```python
from build123d import *

# Parameters (mm, degrees)
IZIM1_R                           = 40.225
Y_KSEKLIK_EKSTR_ZYON1_DEPTH       = 5
IZIM2_W                           = 5
IZIM2_H                           = 15
Y_KSEKLIK_EKSTR_ZYON2_DEPTH       = 64
IZIM3_W                           = 8.48037671
IZIM3_H                           = 5
KES_EKSTR_ZYON1_DEPTH             = 128
IZIM6_R                           = 25
Y_KSEKLIK_EKSTR_ZYON4_DEPTH       = 5
IZIM7_W                           = 5
IZIM7_H                           = 5
Y_KSEKLIK_EKSTR_ZYON5_DEPTH       = 2
IZIM8_W                           = 5
IZIM8_H                           = 5
Y_KSEKLIK_EKSTR_ZYON6_DEPTH       = 7
IZIM9_W                           = 5.33982185
IZIM9_H                           = 8.96327239
KES_EKSTR_ZYON2_DEPTH             = 23
IZIM10_W                          = 16.71
IZIM10_H                          = 5
Y_KSEKLIK_EKSTR_ZYON7_DEPTH       = 15
IZIM13_W                          = 0.39
IZIM13_H                          = 5
Y_KSEKLIK_EKSTR_ZYON9_DEPTH       = 15
Y_KSEKLIK_EKSTR_ZYON10_DEPTH      = 3
Y_KSEKLIK_EKSTR_ZYON10_DEPTH_BACK = 18
IZIM14_W                          = 15
IZIM14_H                          = 5
IZIM11_W                          = 15.71
IZIM11_H                          = 5
Y_KSEKLIK_EKSTR_ZYON11_DEPTH      = 15
Y_KSEKLIK_EKSTR_ZYON12_DEPTH      = 3
Y_KSEKLIK_EKSTR_ZYON12_DEPTH_BACK = 18
IZIM16_W                          = 15
IZIM16_H                          = 5
IZIM17_W                          = 120.128605811
IZIM17_H                          = 27.620146719
KES_EKSTR_ZYON3_DEPTH             = 50
IZIM18_R                          = 5
KES_EKSTR_ZYON4_DEPTH             = 100
IZIM20_R                          = 20
IZIM20_R_2                        = 10
Y_KSEKLIK_EKSTR_ZYON14_DEPTH      = 35
IZIM21_R                          = 10
KES_EKSTR_ZYON5_DEPTH             = 45


with BuildPart() as part:
    # Çizim1 → Yükseklik-Ekstrüzyon1 (new body)
    with BuildSketch(Plane.XY):
        Circle(IZIM1_R)
    extrude(amount=Y_KSEKLIK_EKSTR_ZYON1_DEPTH)

    # Çizim2 → Yükseklik-Ekstrüzyon2 (add, symmetric)
    with BuildSketch(Plane(origin=(0, 0, 0), x_dir=(0, 0, -1), z_dir=(1, 0, 0))):
        with Locations((-2.5, 0)):
            Rectangle(IZIM2_W, IZIM2_H)
    extrude(amount=Y_KSEKLIK_EKSTR_ZYON2_DEPTH, both=True)

    # Çizim3 → Kes-Ekstrüzyon1 (cut)
    with BuildSketch(Plane.XZ.offset(7.5)):
        with Locations((-59.759811645, 2.5)):
            Rectangle(IZIM3_W, IZIM3_H)
    extrude(amount=-KES_EKSTR_ZYON1_DEPTH, mode=Mode.SUBTRACT)

    # Çizim7 → Yükseklik-Ekstrüzyon5 (add)
    with BuildSketch(Plane.XY.offset(5)):
        Polygon((35.024990748, -17.334936491), (30.694863729, -14.834936491), (28.194863729, -19.165063509), (32.524990748, -21.665063509), align=None)
        with Locations((0, 36.5)):
            Rectangle(IZIM7_W, IZIM7_H)
        Polygon((-32.524990748, -21.665063509), (-28.194863729, -19.165063509), (-30.694863729, -14.834936491), (-35.024990748, -17.334936491), align=None)
    extrude(amount=Y_KSEKLIK_EKSTR_ZYON5_DEPTH)


with BuildPart() as body_2:
    # Çizim6 → Yükseklik-Ekstrüzyon4 (new body)
    with BuildSketch(Plane.XY.offset(25)):
        Circle(IZIM6_R)
    extrude(amount=Y_KSEKLIK_EKSTR_ZYON4_DEPTH)

    # Çizim8 → Yükseklik-Ekstrüzyon6 (add)
    with BuildSketch(Plane.XY.offset(30)):
        Polygon((22.034609691, -9.834936491), (17.704482672, -7.334936491), (15.204482672, -11.665063509), (19.534609691, -14.165063509), align=None)
        with Locations((0, 21.5)):
            Rectangle(IZIM8_W, IZIM8_H)
        Polygon((-19.534609691, -14.165063509), (-15.204482672, -11.665063509), (-17.704482672, -7.334936491), (-22.034609691, -9.834936491), align=None)
    extrude(amount=-Y_KSEKLIK_EKSTR_ZYON6_DEPTH)


    add(part.part)  # loft1 joins it to this body
    # loft from a face of the part (loft1)
    loft([body_2.faces().sort_by_distance((-18.619546181, -10.75, 23))[0], body_2.faces().sort_by_distance((-31.609927238, -18.25, 7))[0]])

    # loft from a face of the part (loft3)
    loft([body_2.faces().sort_by_distance((0, 36.5, 7))[0], body_2.faces().sort_by_distance((0, 21.5, 23))[0]])

    # Çizim9 → Kes-Ekstrüzyon2 (cut)
    with BuildSketch(Plane.XZ.offset(7.5)):
        with Locations((62.899534215, 2.077883617)):
            Rectangle(IZIM9_W, IZIM9_H)
    extrude(amount=-KES_EKSTR_ZYON2_DEPTH, mode=Mode.SUBTRACT)

    # Çizim10 → Yükseklik-Ekstrüzyon7 (add)
    with BuildSketch(Plane.XZ.offset(7.5)):
        with Locations((-52.87462329, 2.5)):
            Rectangle(IZIM10_W, IZIM10_H)
    extrude(amount=-Y_KSEKLIK_EKSTR_ZYON7_DEPTH)

    # Çizim13 → Yükseklik-Ekstrüzyon9 (add)
    with BuildSketch(Plane.XZ.offset(7.5)):
        with Locations((-61.42462329, 2.5)):
            Rectangle(IZIM13_W, IZIM13_H)
    extrude(amount=-Y_KSEKLIK_EKSTR_ZYON9_DEPTH)

    # Çizim14 → Yükseklik-Ekstrüzyon10 (add, two sides: drawn at the far end of the back side and taken through both)
    with BuildSketch(Plane.XZ.offset(7.5).offset(-Y_KSEKLIK_EKSTR_ZYON10_DEPTH_BACK)):
        with Locations((-53.40962329, 2.5)):
            Rectangle(IZIM14_W, IZIM14_H)
    extrude(amount=Y_KSEKLIK_EKSTR_ZYON10_DEPTH + Y_KSEKLIK_EKSTR_ZYON10_DEPTH_BACK)

    # Çizim11 → Yükseklik-Ekstrüzyon11 (add)
    with BuildSketch(Plane.XZ.offset(7.5)):
        with Locations((53.76462329, 2.5)):
            Rectangle(IZIM11_W, IZIM11_H)
    extrude(amount=-Y_KSEKLIK_EKSTR_ZYON11_DEPTH)

    # Çizim16 → Yükseklik-Ekstrüzyon12 (add, two sides: drawn at the far end of the back side and taken through both)
    with BuildSketch(Plane.XZ.offset(7.5).offset(-Y_KSEKLIK_EKSTR_ZYON12_DEPTH_BACK)):
        with Locations((53.40962329, 2.5)):
            Rectangle(IZIM16_W, IZIM16_H)
    extrude(amount=Y_KSEKLIK_EKSTR_ZYON12_DEPTH + Y_KSEKLIK_EKSTR_ZYON12_DEPTH_BACK)

    # Çizim17 → Kes-Ekstrüzyon3 (cut, symmetric)
    with BuildSketch(Plane(origin=(0, 0, 0), x_dir=(1, 0, 0), z_dir=(0, 1, 0))):
        with Locations((6.654679615, -18.81007336)):
            Rectangle(IZIM17_W, IZIM17_H)
    extrude(amount=KES_EKSTR_ZYON3_DEPTH, both=True, mode=Mode.SUBTRACT)

    # Çizim18 → Kes-Ekstrüzyon4 (cut)
    with BuildSketch(Plane(origin=(0, 0, 0), x_dir=(-1, 0, 0), z_dir=(0, 0, -1))):
        Circle(IZIM18_R)
    extrude(amount=-KES_EKSTR_ZYON4_DEPTH, mode=Mode.SUBTRACT)

    # Çizim20 → Yükseklik-Ekstrüzyon14 (add)
    with BuildSketch(Plane(origin=(0, 0, 0), x_dir=(-1, 0, 0), z_dir=(0, 0, -1))):
        with Locations(Location((0, 0, 0), (0, 0, 180))):
            Circle(IZIM20_R)
        Circle(IZIM20_R_2, mode=Mode.SUBTRACT)
    extrude(amount=Y_KSEKLIK_EKSTR_ZYON14_DEPTH)

    # Çizim21 → Kes-Ekstrüzyon5 (cut)
    with BuildSketch(Plane(origin=(0, 0, 0), x_dir=(-1, 0, 0), z_dir=(0, 0, -1))):
        with Locations(Location((0, 0, 0), (0, 0, 180))):
            Circle(IZIM21_R)
    extrude(amount=-KES_EKSTR_ZYON5_DEPTH, mode=Mode.SUBTRACT)


solid = body_2.part
```
Model file for the job. Use its own axes, mm. A direction names the side the tool comes from. Give positions to 0.01 mm unless a question says otherwise; leave off trailing zeros. Write each loop counter-clockwise with the first axis right and the second up, starting at its lowest first coordinate (ties: lowest second). Pieces come first, ordered by that corner, then holes. Notation, with made-up numbers: (31, 23.5) - (86, 23.5) arc R15 cw to (86, 29.5) - close; hole circle Ø9 at (71.5, 33). An arc over 180 degrees is marked (long way). One line per question, with ' | ' between items. Start each with the question number.
(1) Wall check: line 1 along Y through (x, z) = (0, -21); line 2 along Y through (x, z) = (0, 2) (3 decimals); line 3 along X through (y, z) = (0.5, -29.5). Give the ranges that are in metal, low to high. Write a range as from..to.
(2) Slice it at B-B on x = 0. Write the cut outline in (y, z) (3 decimals).
(3) Two-plate mould, pull along X, no slides. Class faces 1 (the face through (60.91, -9, 2)), 2 (the face through (-45.91, -9, 2)), 3 (the face through (-5, -9, -35)): +X half, -X half, draft (parallel to the pull), parting line (faces both ways), or undercut.
(4) 3-axis set-ups, long thin cutter, end or side, ignore diameter. For faces 4 (the face through (-43, 7.5, 3)), 5 (the face through (13, 18, 0)), 6 (the face through (-54, -10.5, 3)): which of +Z, -Z, +X, -X, +Y, -Y reach the whole face in a straight line?
(5) Slice it at C-C on z = -19. Write the cut outline in (x, y).
(6) Slice it at A-A on y = 0. Write the cut outline in (x, z), plus the area to 3 significant figures.
(7) Pin check, flat tips, straight feed: P1, Ø0.9, axis at y = 8.5, z = 3.5, coming from the -X side; P2, Ø12, axis at x = 13, z = -13, coming from the +Y side (3 decimals); P3, Ø2.5, axis at x = -52, z = 3.5, coming from the -Y side; P4, Ø3, axis at x = 28.5, y = 30, coming from the +Z side. Stop position of each tip, or through.
(8) Slice it at D-D on x = 41.5. Write the cut outline in (y, z), plus the area to 3 significant figures.
Results below:
1) line 1: -20..-10, 10..20 | line 2: -40.225..-10, 10..40.225 | line 3: -19.99..-9.99, 9.99..19.99
2) outline: (-40.225, 0) - (-20, 0) - (-20, -35) - (-10, -35) - (-10, 5) - (-40.225, 5) - close; (10, -35) - (20, -35) - (20, 0) - (40.225, 0) - (40.225, 5) - (10, 5) - close
3) face 1: +X half | face 2: undercut | face 3: draft
4) face 4: +Z, -Z, +Y | face 5: -Z | face 6: +Z, -Z, -X, -Y
5) outline: circle Ø40 at (0, 0); hole circle Ø20 at (0, 0)
6) outline: (-61.62, 0) - (-20, 0) - (-20, -35) - (-10, -35) - (-10, 5) - (-61.62, 5) - close; (10, -35) - (20, -35) - (20, 0) - (61.62, 0) - (61.62, 5) - (10, 5) - close | area: 1,220 mm^2
7) P1: x = -60.91 | P2: y = 18.735 | P3: y = -10.5 | P4: z = 5
8) outline: (-7.5, 0) - (7.5, 0) - (7.5, 5) - (-7.5, 5) - close | area: 75.0 mm^2
